Input: part model. Units: mm. Frame: model coordinates. Face numbers are marked on the shaded views. A direction names the side the tool comes from. Give positions to 0.01 mm unless a question says otherwise; leave off trailing zeros. Order: outer loops, then holes, each group sorted by start corner. A loop starts at its lowest first (then second) coordinate and runs counter-clockwise, first axis right, second up. Notation, with made-up numbers: (72.25, -23) - (131.25, -23) arc R20 cw to (131.25, -13) - close; hole circle Ø8 at (-9.5, 31.25). An arc over 180 degrees is marked (long way). Use a Markdown table: item, result.
from build123d import *

# Parameters (mm, degrees)
F0_R     = 20
F1_DEPTH = 6
F3_START = 14
F3_DEPTH = 22
F4_R     = 6
F5_DEPTH = 4
F7_COUNT = 3


with BuildPart() as f1:
    # F0 (on Top) → F1 (new body)
    with BuildSketch(Plane.XY):
        Polygon((20.2072594216, 35), (-20.2072594216, 35), (-40.4145188433, 0), (-20.2072594216, -35), (20.2072594216, -35), (40.4145188433, 0), align=None)
        Circle(F0_R, mode=Mode.SUBTRACT)
    extrude(amount=F1_DEPTH)

    # F2 (on Right) → F3 (join)
    with BuildSketch(Plane.YZ.offset(F3_START)):
        Polygon((-29.2928932188, 8), (-32.1213203436, 10.8284271247), (-35, 7.9497474683), (-35, 0), (-17.8076118446, 0), (-17.8076118446, 17.7279220614), (-21.5147186258, 21.4350288425), (-23.6360389693, 19.313708499), (-20.8076118446, 16.4852813742), align=None)
        Polygon((-23.6360389693, 19.313708499), (-32.1213203436, 10.8284271247), (-29.2928932188, 8), (-20.8076118446, 16.4852813742), align=None)
    extrude(amount=F3_DEPTH)

    # F4 (on face) → F5 (cut)
    with BuildSketch(Plane(origin=(0, -21.4748737342, 21.4748737342), x_dir=(1, 0, 0), z_dir=(0, -0.7071067812, 0.7071067812))):
        with Locations((25, -9.0563491861)):
            Circle(F4_R)
    extrude(amount=-F5_DEPTH, mode=Mode.SUBTRACT)

    # F6: F1 across plane


with BuildPart() as f1_1:
    add(f1.part)
    add(f1.part.mirror(Plane.YZ))

    # F7: F1 ×3 about axis
    f7_axis = Axis((0, 0, 0), (0, 0, -1))


with BuildPart() as f1_2:
    add(f1_1.part)
    for i in range(1, F7_COUNT):
        add(f1_1.part.rotate(f7_axis, i * 360 / F7_COUNT))


solid = f1_2.part
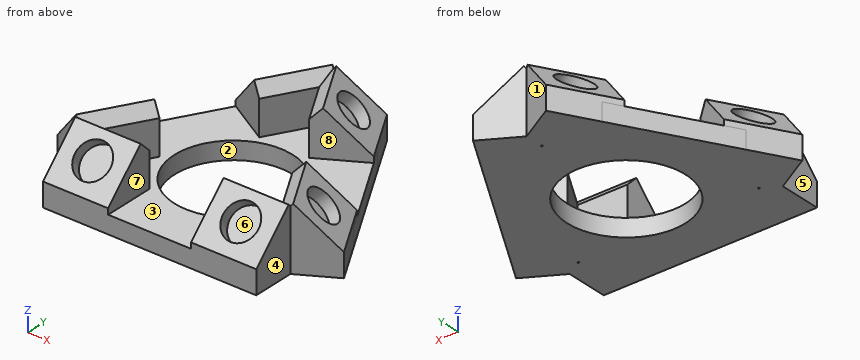
1. Section query B-B (y = 24). Return loops of the section in (x, z).
Response:
| item | result |
|---|---|
| outline | (-26.56, 0) - (26.56, 0) - (26.56, 6) - (13.57, 6) - (13.57, 19.2) - (10.99, 21.44) - (6.71, 17.73) - (6.71, 6) - (-6.71, 6) - (-6.71, 17.73) - (-10.99, 21.44) - (-13.57, 19.2) - (-13.57, 6) - (-26.56, 6) - close |
2. Pin query (flat end, axial travel): pin 1 (6 mm diameter, centred on y = 32.5, z = 10.5, fed in from -X); pin 2 (8.5 mm diameter, centred on x = -20, z = 6.5, fed in from +Y); pin 3 (6 mm diameter, centred on x = 10.5, y = -9.5, fed in from +Z); pin 4 (1 mm diameter, centred on x = -20, y = -25, fed in from +Z). Return the tip coordinate at first contact, or that it passes through.
Response:
| item | result |
|---|---|
| pin 1 | stops at x = -22.56 |
| pin 2 | stops at y = 42.72 |
| pin 3 | passes through |
| pin 4 | stops at z = 18.45 |
3. Set-up query: the marked faces 5, 6, 7 and 8. Return all of +Z, -Z, +X, -X, +Y, -Y with unobstructed straight access to the full face (end or side cutting, diameter ignored); none if empty.
Response:
| item | result |
|---|---|
| face 5 | +Z, -Z, -X, -Y |
| face 6 | none |
| face 7 | +Z, -Y |
| face 8 | +Z, +X |
4. Material intervals for line 1 along X through (y, z) = (0, 3.8); line 2 along Z through (x, y) = (-23, 1.5); line 3 along X through (y, z) = (-24, 16), sorted ascending.
Response:
| item | result |
|---|---|
| line 1 | x = -40.41 to -20, 20 to 40.41 |
| line 2 | z = 0 to 6 |
| line 3 | x = -36 to -29.94, -20.06 to -14, 14 to 20.06, 29.94 to 36 |
5. Mould query, pull axis Y, two halves, no side actions, for the marked faces 1, 2, 3 and 4. Classes: pulls with the +Y half, pulls with the -Y half, needs draft (parallel to the pull), parting line crosses it, or undercut.
Response:
| item | result |
|---|---|
| face 1 | pulls with the +Y half |
| face 2 | undercut |
| face 3 | undercut |
| face 4 | needs draft |
6. Section query A-A (y = 7). Return loops of the section in (x, z) (3 decimals), then the cut area to 3 significant figures.
Response:
| item | result |
|---|---|
| outline | (-36.373, 0) - (-18.735, 0) - (-18.735, 6) - (-36.373, 6) - close; (18.735, 0) - (36.373, 0) - (36.373, 6) - (18.735, 6) - close |
| area | 212 mm^2 |
